Source: CAD feature listing. Evaluate the final solid. Frame: model axes, mm. A direction names the side the tool comes from. Round coordinates to 2 decimals unless told otherwise and drop trailing zeros. Write each loop counter-clockwise with the first axis right and the second up, starting at its lowest first coordinate (ties: lowest second). Pieces come first, ordered by that corner, then holes. Notation, with made-up numbers: M 62,60.5 L 77,60.5 A20 ccw 77,69.5 Z; hole C 45.25,88 d6. An arc over 180 degrees is marked long. Use a Markdown table: item, result.
```python
from build123d import *

# Parameters (mm, degrees)
F0_W     = 3.175
F0_H     = 160.30702
F1_DEPTH = 114.3
F2_W     = 145.818248
F2_H     = 3.175
F3_DEPTH = 12.7
F5_DEPTH = 25.4
F7_DEPTH = 25.4


with BuildPart() as f1:
    # F0 (on Top) → F1 (new body)
    with BuildSketch(Plane.XY):
        Rectangle(F0_W, F0_H)
    extrude(amount=F1_DEPTH)

    # F2 (on face) → F3 (join)
    with BuildSketch(Plane.YZ.offset(1.5875)):
        with Locations((-7.244386, 112.7125)):
            Rectangle(F2_W, F2_H)
    extrude(amount=F3_DEPTH)

    # F4 (on face) → F5 (cut)
    with BuildSketch(Plane.XY.offset(114.3)):
        Polygon((14.2875, 65.664738), (1.5875, 65.664738), (14.2875, 60.06493), align=None)
        Polygon((1.5875, -80.15351), (14.2875, -80.15351), (14.2875, -66.047616), align=None)
    extrude(amount=-F5_DEPTH, mode=Mode.SUBTRACT)

    # F6 (on face) → F7 (cut)
    with BuildSketch(Plane.XY.offset(114.3)):
        with BuildLine():
            ThreePointArc((11.1125, 50.164834), (10.182564, 52.409898), (7.9375, 53.339834))
            Line((7.9375, 53.339834), (7.9375, 46.989834))
            ThreePointArc((7.9375, 46.989834), (10.182564, 47.91977), (11.1125, 50.164834))
        make_face()
        with BuildLine():
            ThreePointArc((11.1125, -60.400563), (10.182564, -58.155499), (7.9375, -57.225563))
            Line((7.9375, -57.225563), (7.9375, -63.575563))
            ThreePointArc((7.9375, -63.575563), (10.182564, -62.645627), (11.1125, -60.400563))
        make_face()
        with BuildLine():
            Line((7.9375, -63.575563), (7.9375, -57.225563))
            ThreePointArc((7.9375, -57.225563), (4.7625, -60.400563), (7.9375, -63.575563))
        make_face()
        with BuildLine():
            ThreePointArc((11.1125, 0), (10.182564, 2.245064), (7.9375, 3.175))
            Line((7.9375, 3.175), (7.9375, -3.175))
            ThreePointArc((7.9375, -3.175), (10.182564, -2.245064), (11.1125, 0))
        make_face()
        with BuildLine():
            Line((7.9375, -3.175), (7.9375, 3.175))
            ThreePointArc((7.9375, 3.175), (4.7625, 0), (7.9375, -3.175))
        make_face()
        with BuildLine():
            Line((7.9375, 46.989834), (7.9375, 53.339834))
            ThreePointArc((7.9375, 53.339834), (4.7625, 50.164834), (7.9375, 46.989834))
        make_face()
    extrude(amount=-F7_DEPTH, mode=Mode.SUBTRACT)


solid = f1.part
```
Q1. Line query: L1, parallel to X at y = 5.5, z = 25.5; L2, parallel to Z at x = 6, y = -14.5 (3 decimals). Output: solid intervals per line, ascending.
Results are:
| item | result |
|---|---|
| L1 | -1.59 to 1.59 |
| L2 | 111.125 to 114.3 |
Q2. First-contact query: pin 1 Ø1 at (x, y) = (5, -33) entering from -Z (3 decimals); pin 2 Ø10 at (y, z) = (-13.5, 19) entering from +X. Flat tips, straight axial feed; report the tip coordinate or a pass-through.
Results are:
| item | result |
|---|---|
| pin 1 | z = 111.125 |
| pin 2 | x = 1.59 |
Q3. Section A-A on y = -25.5. Return loops of the section in (x, z) (1 decimal).
Results are:
| item | result |
|---|---|
| outline | M -1.6,0 L 1.6,0 L 1.6,111.1 L 14.3,111.1 L 14.3,114.3 L -1.6,114.3 Z |
Q4. Section B-B on z = 79.5. Return loops of the section in (x, y).
Results are:
| item | result |
|---|---|
| outline | M -1.59,-80.15 L 1.59,-80.15 L 1.59,80.15 L -1.59,80.15 Z |
Q5. Reachability of faces 1 (the flat face through (-1.588, -1, 56)), 2 (the flat face through (8, -8, 111.125)) from +Z, -Z, +X, -X, +Y, -Y: full face, straight path, thin tool, end or side. Return the list, or none.
Results are:
| item | result |
|---|---|
| face 1 | +Z, -Z, -X, +Y, -Y |
| face 2 | -Z, +X, +Y, -Y |
